Autodesk Inventor part; units mm, degrees
ref_plane "YZ Plane" through (0, 0, 0) normal (1, 0, 0) x (0, 1, 0)
ref_plane "XZ Plane" through (0, 0, 0) normal (0, 1, 0) x (-1, 0, 0)
ref_plane "XY Plane" through (0, 0, 0) normal (0, 0, 1) x (1, 0, 0)
sketch "Sketch1" plane through (0, 0, 0) normal (0, 0, 1) x (1, 0, 0)
  line L0 (0, 0) -> (150, 0)
  line L1 (150, 0) -> (150, 80)
  line L2 (150, 80) -> (0, 80)
  line L3 (0, 80) -> (0, 0)
  dimension "d0" = 150
  dimension "d1" = 80
extrude "Extrusion1" add sketch "Sketch1" along normal blind 5
sketch "Sketch2" plane through (0, 0, 5) normal (0, 0, 1) x (1, 0, 0)
  line L0 (0, 0) -> (150, 0)
  line L1 (150, 80) -> (0, 80)
  line L2 (129, 0) -> (21, 0)
  line L3 (21, 0) -> (21, 80)
  line L4 (21, 80) -> (129, 80)
  line L5 (129, 80) -> (129, 0)
  line L6 (126, 3) -> (24, 3)
  line L7 (24, 3) -> (24, 77)
  line L8 (24, 77) -> (126, 77)
  line L9 (126, 77) -> (126, 3)
  line L10 (150, 0) -> (150, 80)
  point P0 (129, 80)
  point P1 (21, 0)
  dimension "d4" = 108
  dimension "d5" = 102
  dimension "d6" = 3
  dimension "d7" = 3
  dimension "d8" = 3
  dimension "d9" = 21
extrude "Extrusion2" add sketch "Sketch2" along normal blind 30 contours L3 L1 L5 L0
chamfer "Chamfer1" distance 2 angle 45 1 edges at (75, 3, 35)
chamfer "Chamfer2" distance 2 angle 45 1 edges at (126, 40, 35)
chamfer "Chamfer3" distance 2 angle 45 2 edges at (75, 77, 35) (24, 40, 35)
sketch "Sketch3" plane through (0, 0, 5) normal (0, 0, 1) x (1, 0, 0)
  circle A0 centre (137.5, 15) radius 3.25
  circle A1 centre (137.5, 65) radius 3.25
  line L0 (150, 0) -> (150, 80)
  line L1 (129, 0) -> (150, 0)
  line L2 (75, -16.6248) -> (75, 70.7208)
  line L3 (0, 80) -> (0, 0)
  circle A2 centre (12.5, 15) radius 3.25
  circle A3 centre (12.5, 65) radius 3.25
  dimension "d21" = 6.5
  dimension "d22" = 6.5
  dimension "d23" = 12.5
  dimension "d24" = 12.5
  dimension "d25" = 50
  dimension "d26" = 15
  dimension "d27" = 75
extrude "Extrusion3" cut sketch "Sketch3" against normal blind 60
properties part number "MediumHolder"
Could you check a few things on this model? Use its own coordinates, in mm. A direction names the side the tool comes from. Give positions to 0.01 mm unless a question says otherwise; leave off trailing zeros. Write each loop counter-clockwise with the first axis right and the second up, starting at its lowest first coordinate (ties: lowest second). Pieces come first, ordered by that corner, then holes. Notation, with made-up numbers: (49, 73.5) - (65, 73.5) arc R27 ccw to (65, 89.5) - close; hole circle Ø3 at (54.25, 21.25). An arc over 180 degrees is marked (long way). One line per item, written item: value. Start each with the question number.
Item 1: Imagine slicing it at A-A, the plane y = 65. List the corners of the cut face in (x, z) for me, and give its area (3 significant figures).
Item 2: I'm going to push flat-ended pins straight in: pin 1 (6.5 mm diameter, centred on x = 141.5, y = 47, fed in from +Z); pin 2 (1.5 mm diameter, centred on y = 69, z = 25, fed in from -X); pin 3 (15 mm diameter, centred on y = 35, z = 13, fed in from +X). Where does each tip first touch, or does it pass through?
Item 3: Imagine slicing it at C-C, the plane x = 12.5. List the corners of the cut face in (y, z) for me.
Item 4: Please list where these lines run through material, in increasing order: line 1 (Y direction, x = 137.5, z = 3.9); line 2 (Y direction, x = 85.5, z = 15); line 3 (X direction, y = 49.5, z = 29). Write a range as from..to.
Item 5: If we mould it in two halves opening along X, with no side actions, what happens to faces 5 (the face through (139, 41, 5)), 6 (the face through (140.502, 63.755, 2.535)), 7 (the face through (150, 39, 2))? For each: +X half, -X half, draft (parallel to the pull), parting line (faces both ways), or undercut.
Item 6: Imagine slicing it at B-B, the plane z = 26. List the corners of the cut face in (x, y) for me, and give its area (3 significant figures).
Item 7: Which directions (+Z, -Z, +X, -X, +Y, -Y) give clear straight access to the entire face, cutting with the end or side of a thin tool? Please do faces 1 (the face through (76, 3, 19)), 2 (the face through (129, 41, 20)), 3 (the face through (21, 39, 20)), 4 (the face through (74, 41, 0)).
Item 8: Imagine slicing it at D-D, the plane y = 21. List the corners of the cut face in (x, z) for me, and give its area (3 significant figures).
Geometry says:
1. outline: (0, 0) - (9.25, 0) - (9.25, 5) - (0, 5) - close; (15.75, 0) - (134.25, 0) - (134.25, 5) - (129, 5) - (129, 35) - (128, 35) - (126, 33) - (126, 5) - (24, 5) - (24, 33) - (22, 35) - (21, 35) - (21, 5) - (15.75, 5) - close; (140.75, 0) - (150, 0) - (150, 5) - (140.75, 5) - close
1. area: 861 mm^2
2. pin 1: z = 5
2. pin 2: x = 21
2. pin 3: x = 129
3. outline: (0, 0) - (11.75, 0) - (11.75, 5) - (0, 5) - close; (18.25, 0) - (61.75, 0) - (61.75, 5) - (18.25, 5) - close; (68.25, 0) - (80, 0) - (80, 5) - (68.25, 5) - close
4. line 1: 0..11.75, 18.25..61.75, 68.25..80
4. line 2: 0..3, 77..80
4. line 3: 21..24, 126..129
5. face 5: draft
5. face 6: undercut
5. face 7: +X half
6. outline: (21, 0) - (129, 0) - (129, 80) - (21, 80) - close; hole (24, 3) - (126, 3) - (126, 77) - (24, 77) - close
6. area: 1,090 mm^2
7. face 1: +Z
7. face 2: +Z, +X, +Y, -Y
7. face 3: +Z, -X, +Y, -Y
7. face 4: -Z, +X, -X, +Y, -Y
8. outline: (0, 0) - (150, 0) - (150, 5) - (129, 5) - (129, 35) - (128, 35) - (126, 33) - (126, 5) - (24, 5) - (24, 33) - (22, 35) - (21, 35) - (21, 5) - (0, 5) - close
8. area: 926 mm^2
